Could you check a few things on this model? Use its own coordinates, in mm. Face numbers are marked on the shaded views. Give positions to 0.01 mm unless a question says otherwise; leave off trailing zeros. Loops run counter-clockwise (first coordinate to the right, second up) from the corner with the lowest first, then second, coordinate; pieces in that order, holes last.
1. Imagine slicing it at B-B (y = -9.5). List the corners of the cut face in (x, z) for me, plus the area to 3 significant figures.
2. Imagine slicing it at A-A (z = 14.75). Count the separate pieces of the cut face and the enclosed holes in it, plus the area to 3 significant figures.
3. For P1, Ø10, axis at x = 82, y = -64, coming from the +Z side; P2, Ø5, axis at x = 44.5, y = -65.5, coming from the +Z side, each with a flat end and sliding along its axis, tell me the tip position at first contact or that it passes through.
4. Imagine slicing it at D-D (y = -51). List the corners of the cut face in (x, z) for me.
5. Imagine slicing it at C-C (x = 54.5). List the corners of the cut face in (y, z) for me, plus the area to 3 significant figures.
6. Thinking about a two-plate mould opening in Y: for the marked faces 1, 2, 3 and 4, which applies, +Y half, -Y half, draft (parallel to the pull), parting line (faces both ways), or undercut?
7. I need wall thicknesses on line 1 along Y through (x, z) = (96.52, 8.5); line 2 along X through (y, z) = (-71.12, 7.5); line 3 along Y through (x, z) = (13.5, 20.75). Which ranges of each line are inside material? Lowest first, please.
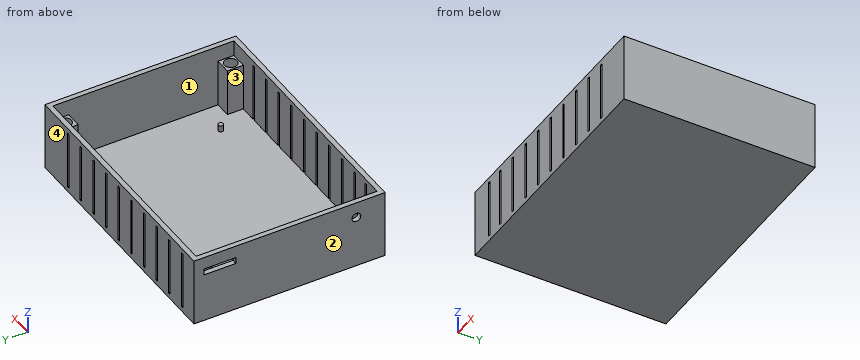
```python
from build123d import *

# Parameters (mm, degrees)
SKETCH16_W          = 101.6
SKETCH16_H          = 76.2
BOSS_EXTRUDE4_DEPTH = 2
SKETCH17_W          = 101.6
SKETCH17_H          = 76.2
SKETCH17_W_2        = 97.6
SKETCH17_H_2        = 72.2
BOSS_EXTRUDE5_DEPTH = 25.4
SKETCH18_R          = 1
BOSS_EXTRUDE6_DEPTH = 2.54
SKETCH19_W          = 1
SKETCH19_H          = 23.4
CUT_EXTRUDE6_DEPTH  = 2
SKETCH20_W          = 1
SKETCH20_H          = 23.4
CUT_EXTRUDE7_DEPTH  = 2
SKETCH21_R          = 1.75
SKETCH21_W          = 2.54
SKETCH21_H          = 12.7
CUT_EXTRUDE8_DEPTH  = 2
SKETCH33_W          = 6.35
SKETCH33_H          = 6.35
SKETCH33_R          = 2.54
BOSS_EXTRUDE7_DEPTH = 19.05


with BuildPart() as part:
    # Sketch16 → Boss-Extrude4 (new body)
    with BuildSketch(Plane.XY):
        with Locations((50.8, -38.1)):
            Rectangle(SKETCH16_W, SKETCH16_H)
    extrude(amount=BOSS_EXTRUDE4_DEPTH)

    # Sketch17 → Boss-Extrude5 (add)
    with BuildSketch(Plane.XY.offset(2)):
        with Locations((50.8, -38.1)):
            Rectangle(SKETCH17_W, SKETCH17_H)
        with Locations((50.8, -38.1)):
            Rectangle(SKETCH17_W_2, SKETCH17_H_2, mode=Mode.SUBTRACT)
    extrude(amount=BOSS_EXTRUDE5_DEPTH)

    # Sketch18 → Boss-Extrude6 (add)
    with BuildSketch(Plane.XY.offset(2)):
        with Locations((14.7, -14.7)):
            Circle(SKETCH18_R)
        with Locations((86.9, -14.7)):
            Circle(SKETCH18_R)
        with Locations((86.9, -61.5)):
            Circle(SKETCH18_R)
        with Locations((14.7, -61.5)):
            Circle(SKETCH18_R)
    extrude(amount=BOSS_EXTRUDE6_DEPTH)

    # Sketch19 → Cut-Extrude6 (cut)
    with BuildSketch(Plane.XZ.offset(76.2)):
        with Locations((9.66, 13.7)):
            Rectangle(SKETCH19_W, SKETCH19_H)
        with Locations((17.28, 13.7)):
            Rectangle(SKETCH19_W, SKETCH19_H)
        with Locations((25.9, 13.7)):
            Rectangle(SKETCH19_W, SKETCH19_H)
        with Locations((34.52, 13.7)):
            Rectangle(SKETCH19_W, SKETCH19_H)
        with Locations((43.14, 13.7)):
            Rectangle(SKETCH19_W, SKETCH19_H)
        with Locations((51.76, 13.7)):
            Rectangle(SKETCH19_W, SKETCH19_H)
        with Locations((60.38, 13.7)):
            Rectangle(SKETCH19_W, SKETCH19_H)
        with Locations((69, 13.7)):
            Rectangle(SKETCH19_W, SKETCH19_H)
        with Locations((77.62, 13.7)):
            Rectangle(SKETCH19_W, SKETCH19_H)
        with Locations((86.24, 13.7)):
            Rectangle(SKETCH19_W, SKETCH19_H)
    extrude(amount=-CUT_EXTRUDE6_DEPTH, mode=Mode.SUBTRACT)

    # Sketch20 → Cut-Extrude7 (cut)
    with BuildSketch(Plane(origin=(0, 0, 0), x_dir=(1, 0, 0), z_dir=(0, 1, 0))):
        with Locations((8.12, -13.7)):
            Rectangle(SKETCH20_W, SKETCH20_H)
        with Locations((16.74, -13.7)):
            Rectangle(SKETCH20_W, SKETCH20_H)
        with Locations((25.36, -13.7)):
            Rectangle(SKETCH20_W, SKETCH20_H)
        with Locations((33.98, -13.7)):
            Rectangle(SKETCH20_W, SKETCH20_H)
        with Locations((42.6, -13.7)):
            Rectangle(SKETCH20_W, SKETCH20_H)
        with Locations((51.22, -13.7)):
            Rectangle(SKETCH20_W, SKETCH20_H)
        with Locations((59.84, -13.7)):
            Rectangle(SKETCH20_W, SKETCH20_H)
        with Locations((68.46, -13.7)):
            Rectangle(SKETCH20_W, SKETCH20_H)
        with Locations((85.7, -13.7)):
            Rectangle(SKETCH20_W, SKETCH20_H)
        with Locations((77.08, -13.7)):
            Rectangle(SKETCH20_W, SKETCH20_H)
    extrude(amount=-CUT_EXTRUDE7_DEPTH, mode=Mode.SUBTRACT)

    # Sketch21 → Cut-Extrude8 (cut)
    with BuildSketch(Plane.ZY):
        with Locations(Location((21.05, -64.77, 0), (0, 0, 270))):
            Circle(SKETCH21_R)
        with Locations((21.13, -10.35)):
            Rectangle(SKETCH21_W, SKETCH21_H)
    extrude(amount=-CUT_EXTRUDE8_DEPTH, mode=Mode.SUBTRACT)

    # Sketch33 → Boss-Extrude7 (add)
    # profile 1 of 4: a face of its own
    with BuildSketch(Plane.XY.offset(2)):
        with Locations((5.175, -5.175)):
            Rectangle(SKETCH33_W, SKETCH33_H)
        with Locations(Location((5.08, -5.08, 0), (0, 0, 180))):
            Circle(SKETCH33_R, mode=Mode.SUBTRACT)
    # profile 2 of 4: a face of its own
    with BuildSketch(Plane.XY.offset(2)):
        with Locations((96.425, -5.175)):
            Rectangle(SKETCH33_W, SKETCH33_H)
        with Locations(Location((96.52, -5.08, 0), (0, 0, 180))):
            Circle(SKETCH33_R, mode=Mode.SUBTRACT)
    # profile 3 of 4: a face of its own
    with BuildSketch(Plane.XY.offset(2)):
        with Locations((5.175, -71.025)):
            Rectangle(SKETCH33_W, SKETCH33_H)
        with Locations(Location((5.08, -71.12, 0), (0, 0, 180))):
            Circle(SKETCH33_R, mode=Mode.SUBTRACT)
    # profile 4 of 4: a face of its own
    with BuildSketch(Plane.XY.offset(2)):
        with Locations((96.425, -71.025)):
            Rectangle(SKETCH33_W, SKETCH33_H)
        with Locations(Location((96.52, -71.12, 0), (0, 0, 180))):
            Circle(SKETCH33_R, mode=Mode.SUBTRACT)
    extrude(amount=BOSS_EXTRUDE7_DEPTH)


solid = part.part
```
Derived:
1. outline: (0, 0) - (101.6, 0) - (101.6, 27.4) - (99.6, 27.4) - (99.6, 2) - (2, 2) - (2, 19.86) - (0, 19.86) - close; (0, 22.4) - (2, 22.4) - (2, 27.4) - (0, 27.4) - close
1. area: 300 mm2
2. separate pieces: 20
2. enclosed holes: 4
2. area: 735 mm2
3. P1: stops at z = 4.54
3. P2: stops at z = 2
4. outline: (0, 0) - (101.6, 0) - (101.6, 27.4) - (99.6, 27.4) - (99.6, 2) - (2, 2) - (2, 27.4) - (0, 27.4) - close
5. outline: (-76.2, 0) - (0, 0) - (0, 27.4) - (-2, 27.4) - (-2, 2) - (-74.2, 2) - (-74.2, 27.4) - (-76.2, 27.4) - close
5. area: 254 mm2
6. face 1: undercut
6. face 2: draft
6. face 3: undercut
6. face 4: +Y half
7. line 1: y = -76.2 to -73.66, -68.58 to -67.85, -8.35 to -7.62, -2.54 to 0
7. line 2: x = 0 to 2.54, 7.62 to 8.35, 93.25 to 93.98, 99.06 to 101.6
7. line 3: y = -76.2 to -74.2, -2 to 0
